Check sheet for the drawn part. Datum: minimum x, y, z corner. Units: mm. A direction names the side the tool comes from. Give positions to 0.01 mm unless a question says otherwise; leave off trailing zeros. Write each loop counter-clockwise with the first axis right and the second up, starting at its lowest first coordinate (ties: lowest second). Pieces come first, ordered by that corner, then holes. Notation, with made-up numbers: (40.25, 8) - (50.25, 8) arc R32 ccw to (50.25, 45) - close; hole circle Ø3 at (83.25, -30.5). An arc over 180 degrees is marked (long way). Answer as a JSON object with one key per item and string values. Group by question number.
Item 1: Sectioned sample at A-A, the plane x = 8. Record the boundary of the cut face in (y, z).
Item 2: Scan lines: line 1 along X through (y, z) = (7.25, 2.5) (1 decimal); line 2 along Y through (x, z) = (2.75, 9.75); line 3 along Y through (x, z) = (12, 3.75). Record each from-to range of solid material in increasing order. Write a range as [from, to].
Item 3: Sectioned sample at C-C, the plane y = 1.5. Record the boundary of the cut face in (x, z), and give its area (3 significant figures).
Item 4: Sectioned sample at B-B, the plane y = 3.55. Record the boundary of the cut face in (x, z).
Item 5: Draft check along Y on the marked faces 1, 2 and 3. Enter one of: +Y half, -Y half, draft (parallel to the pull), parting line (faces both ways), or undercut.
Item 6: Tool access check on the marked faces 4, 5 and 6. Record the directions out of +Z, -Z, +X, -X, +Y, -Y that give a thin tool (end or side, any length) a straight path to the whole face; none if there is none.
Item 7: Go/stop test with flat-tipped pins: pin 1 (1.1 mm diameter, centred on x = 2.29, z = 6.15, fed in from +Y); pin 2 (8 mm diameter, centred on y = 3.5, z = 4, fed in from -X); pin 3 (1.4 mm diameter, centred on x = 6.15, z = 2.29, fed in from +Y); pin 4 (2 mm diameter, centred on x = 8.5, z = 5.5, fed in from +Y). Record where each tip stops, or that it passes through.
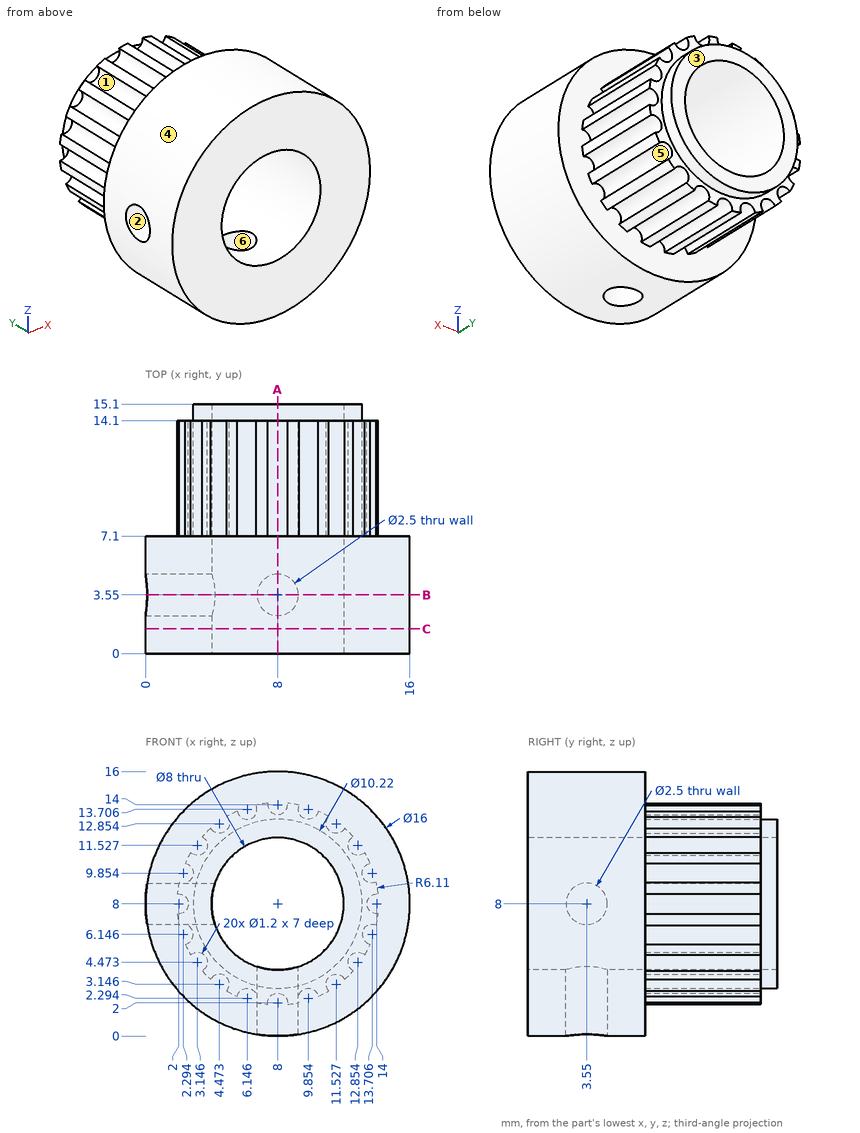
Geometry check:
{
 "1": {"outline": "(0, 0) - (2.3, 0) - (2.3, 4) - (0, 4) - close; (0, 12) - (15.1, 12) - (15.1, 13.11) - (14.1, 13.11) - (14.1, 13.4) - (7.1, 13.4) - (7.1, 16) - (0, 16) - close; (4.8, 0) - (7.1, 0) - (7.1, 2.6) - (14.1, 2.6) - (14.1, 2.89) - (15.1, 2.89) - (15.1, 4) - (4.8, 4) - close"},
 "2": {"line 1": "[5.3, 5.6], [6.7, 7.7], [8.3, 9.3], [10.4, 10.7]", "line 2": "[0, 7.1]", "line 3": "[0, 14.1]"},
 "3": {"outline": "circle Ø16 at (8, 8); hole circle Ø8 at (8, 8)", "area": "151 mm^2"},
 "4": {"outline": "(0.1, 6.75) arc R8 ccw to (6.75, 0.1) - (6.75, 4.2) arc R4 cw to (4.2, 6.75) - close; (0.1, 9.25) - (4.2, 9.25) arc R4 cw (long way) to (9.25, 4.2) - (9.25, 0.1) arc R8 ccw (long way) to start"},
 "5": {"face 1": "draft", "face 2": "undercut", "face 3": "+Y half"},
 "6": {"face 4": "+Y, -Y", "face 5": "+Y", "face 6": "-Z"},
 "7": {"pin 1": "y = 7.1", "pin 2": "x = 0", "pin 3": "y = 14.1", "pin 4": "through"}
}
